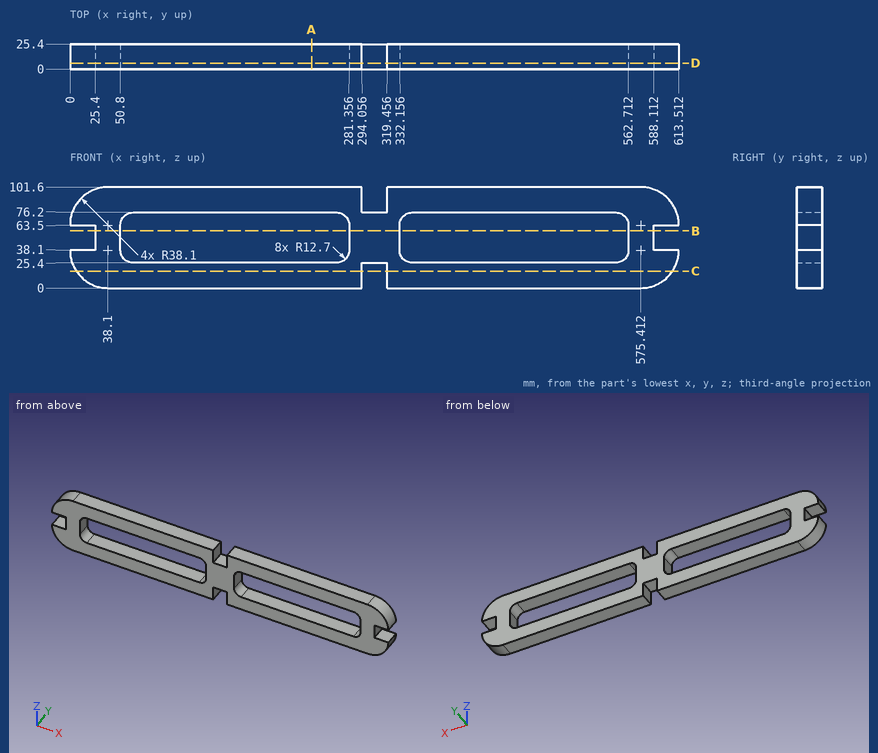
Geometry: see drawing. Coordinates: mm, zero at the bounding-box minimum. Round coordinates to 2 decimals unless told otherwise and drop trailing zeros. Write each loop counter-clockwise with the first axis right and the second up, starting at its lowest first coordinate (ties: lowest second). Pieces come first, ordered by that corner, then holes.
Item 1: Section query B-B (z = 57.5). Return loops of the section in (x, y) (1 decimal), plus the area to 3 significant figures.
Item 2: Section query D-D (y = 6). Give the number of separate pieces and of enclosed holes in the cut face, plus the area to 3 significant figures.
Item 3: Section query A-A (x = 243.5). Return loops of the section in (y, z).
Item 4: Material intervals for L1, parallel to X at y = 10.5, z = 46.5 (1 decimal); L2, parallel to X at y = 13, z = 36.5 (1 decimal); L3, parallel to Z at x = 98, y = 20.25, sorted ascending.
Item 5: Section query C-C (z = 17). Return loops of the section in (x, y) (1 decimal).
Item 6: Pin query (flat end, axial travel): P1, Ø12, axis at y = 10.5, z = 18, coming from the -X side (1 decimal); P2, Ø7.5, axis at y = 13.5, z = 46, coming from the -X side; P3, Ø12.5, axis at y = 12.5, z = 19, coming from the +X side. Return the tip coordinate at first contact, or that it passes through.
Completed:
1. outline: (25.4, 0) - (50.8, 0) - (50.8, 25.4) - (25.4, 25.4) - close; (281.4, 0) - (332.2, 0) - (332.2, 25.4) - (281.4, 25.4) - close; (562.7, 0) - (588.1, 0) - (588.1, 25.4) - (562.7, 25.4) - close
1. area: 2,580 mm2
2. separate pieces: 1
2. enclosed holes: 2
2. area: 35,400 mm2
3. outline: (0, 0) - (25.4, 0) - (25.4, 25.4) - (0, 25.4) - close; (0, 76.2) - (25.4, 76.2) - (25.4, 101.6) - (0, 101.6) - close
4. L1: x = 25.4 to 50.8, 281.4 to 332.2, 562.7 to 588.1
4. L2: x = 0 to 50.9, 281.3 to 332.3, 562.6 to 613.5
4. L3: z = 0 to 25.4, 76.2 to 101.6
5. outline: (6.4, 0) - (294.1, 0) - (294.1, 25.4) - (6.4, 25.4) - close; (319.5, 0) - (607.1, 0) - (607.1, 25.4) - (319.5, 25.4) - close
6. P1: stops at x = 2.7
6. P2: stops at x = 25.4
6. P3: stops at x = 611.28
